from build123d import *

# Parameters (mm, degrees)
SKETCH1_W           = 25.4
SKETCH1_H           = 25.4
SKETCH1_W_2         = 20.32
SKETCH1_H_2         = 20.32
BOSS_EXTRUDE1_DEPTH = 222.25
SKETCH2_R           = 6.35
SKETCH2_R_2         = 3.175
CUT_EXTRUDE1_DEPTH  = 222.25
SKETCH4_W           = 76.2
SKETCH4_H           = 101.6
BOSS_EXTRUDE3_DEPTH = 6.35


with BuildPart() as part:
    # Sketch1 → Boss-Extrude1 (new body)
    with BuildSketch(Plane(origin=(0, 0, 0), x_dir=(1, 0, 0), z_dir=(0, 1, 0))):
        Rectangle(SKETCH1_W, SKETCH1_H)
        Rectangle(SKETCH1_W_2, SKETCH1_H_2, mode=Mode.SUBTRACT)
    extrude(amount=BOSS_EXTRUDE1_DEPTH)

    # Sketch2 → Cut-Extrude1 (cut)
    with BuildSketch(Plane.XY.offset(12.7)):
        with Locations((0, 209.55)):
            Circle(SKETCH2_R)
        with Locations((0, 6.35)):
            Circle(SKETCH2_R_2)
        with Locations((0, 88.9)):
            Circle(SKETCH2_R_2)
    extrude(amount=-CUT_EXTRUDE1_DEPTH, mode=Mode.SUBTRACT)

    # Sketch4 → Boss-Extrude3 (add)
    with BuildSketch(Plane.ZY.offset(12.7)):
        with Locations((0, 50.8)):
            Rectangle(SKETCH4_W, SKETCH4_H)
    extrude(amount=BOSS_EXTRUDE3_DEPTH)


solid = part.part
CAD build for the part. Positions are in the model's coordinates, mm. A direction names the side the tool comes from. Round coordinates to 2 decimals unless told otherwise and drop trailing zeros. Write each loop counter-clockwise with the first axis right and the second up, starting at its lowest first coordinate (ties: lowest second). Pieces come first, ordered by that corner, then holes. Notation, with made-up numbers: M -4,5.25 L 30,5.25 A22 ccw 30,42.25 Z; hole C -22,65 d9. An arc over 180 degrees is marked long. Put each result on its own line as item: value. Start each with the question number.
1) 3-axis set-ups, long thin cutter, end or side, ignore diameter. For faces 4 (the cylindrical face through (-0.69, 85.8, -11.41)), 5 (the flat face through (-10.16, 110, 0)), 6 (the flat face through (-12.7, 52, 25)), 7 (the flat face through (-16, 101.6, -1)), 8 (the flat face through (0, 110, -12.7)): which of +Z, -Z, +X, -X, +Y, -Y reach the whole face in a straight line?
2) Pull direction Y, two halves, no side cores. Call faces 1 (the flat face through (-16, 50, -38.1)), 2 (the cylindrical face through (-0.69, 85.8, 11.45)), 3 (the flat face through (-13, 0, 0)): pulls with the +Y half, pulls with the -Y half, needs draft (parallel to the pull), parting line crosses it, or undercut.
3) Saw through at D-D, the plane z = -23. Write the cut outline in (x, y).
4) Pin check, flat tips, straight feed: pin 1 Ø10 at (x, z) = (-8.5, -29) entering from +Y; pin 2 Ø12 at (x, y) = (4, 85.5) entering from +Z; pin 3 Ø7.5 at (y, z) = (170, -3.5) entering from -X. Stop position of each tip, or through.
5) Drill centre lines: probe 1 along Y at (x, z) = (0, 12) (3 decimals); probe 2 along Z at (x, y) = (-5, 36.5); probe 3 along X at (y, z) = (59, 2). Where is each one in solid material? Low to high. Write a range as [from, to].
6) Saw through at B-B, the plane y = 161. Write the cut outline in (x, z), and give its area (3 significant figures).
7) Saw through at C-C, the plane z = 3. Write the cut outline in (x, y).
8) Saw through at A-A, the plane y = 6.35. Write the cut outline in (x, z) (3 decimals), and give its area (3 significant figures).
Resolved:
1. face 4: +Z, -Z
1. face 5: +Y, -Y
1. face 6: +Z, +X, +Y, -Y
1. face 7: +Z, -Z, -X, +Y
1. face 8: -Z, +X, +Y, -Y
2. face 1: needs draft
2. face 2: undercut
2. face 3: pulls with the -Y half
3. outline: M -19.05,0 L -12.7,0 L -12.7,101.6 L -19.05,101.6 Z
4. pin 1: y = 101.6
4. pin 2: z = 12.7
4. pin 3: x = -12.7
5. probe 1: [0, 3.175], [9.525, 85.725], [92.075, 203.2], [215.9, 222.25]
5. probe 2: [-12.7, -10.16], [10.16, 12.7]
5. probe 3: [-19.05, -10.16], [10.16, 12.7]
6. outline: M -12.7,-12.7 L 12.7,-12.7 L 12.7,12.7 L -12.7,12.7 Z; hole M -10.16,-10.16 L 10.16,-10.16 L 10.16,10.16 L -10.16,10.16 Z
6. area: 232 mm²
7. outline: M -19.05,0 L -10.16,0 L -10.16,222.25 L -12.7,222.25 L -12.7,101.6 L -19.05,101.6 Z; M 10.16,0 L 12.7,0 L 12.7,222.25 L 10.16,222.25 Z
8. outline: M -19.05,-38.1 L -12.7,-38.1 L -12.7,-12.7 L -3.175,-12.7 L -3.175,-10.16 L -10.16,-10.16 L -10.16,10.16 L -3.175,10.16 L -3.175,12.7 L -12.7,12.7 L -12.7,38.1 L -19.05,38.1 Z; M 3.175,-12.7 L 12.7,-12.7 L 12.7,12.7 L 3.175,12.7 L 3.175,10.16 L 10.16,10.16 L 10.16,-10.16 L 3.175,-10.16 Z
8. area: 684 mm²
